from build123d import *

# Parameters (mm, degrees)
SKETCH1_W                = 20
SKETCH1_H                = 60
BOSS_EXTRUDE1_DEPTH      = 15
SKETCH2_W                = 10.25
SKETCH2_H                = 10.1
CUT_EXTRUDE1_DEPTH       = 1
CUT_EXTRUDE1_DEPTH_BACK  = 21
SKETCH3_R                = 4.15
CUT_EXTRUDE2_DEPTH       = 16
BOSS_EXTRUDE2_DEPTH      = 2.5
BOSS_EXTRUDE2_DEPTH_BACK = 22.5
CHAMFER1_SIZE            = 1
CHAMFER1_SIZE2           = 0.577350269
CHAMFER1_PART_2_SIZE     = 1
CHAMFER1_PART_2_SIZE2    = 0.577350269


with BuildPart() as part:
    # Sketch1 → Boss-Extrude1 (new body)
    with BuildSketch(Plane(origin=(0, 0, 0), x_dir=(1, 0, 0), z_dir=(0, 1, 0))):
        Rectangle(SKETCH1_W, SKETCH1_H)
    extrude(amount=BOSS_EXTRUDE1_DEPTH)

    # Sketch2 → Cut-Extrude1 (cut, two sides)
    with BuildSketch(Plane(origin=(10, 0, 0), x_dir=(0, 0, -1), z_dir=(1, 0, 0))) as cut_extrude1_sk:
        with Locations((0, 5.05)):
            Rectangle(SKETCH2_W, SKETCH2_H)
    extrude(amount=CUT_EXTRUDE1_DEPTH, mode=Mode.SUBTRACT)
    extrude(cut_extrude1_sk.sketch, amount=-CUT_EXTRUDE1_DEPTH_BACK, mode=Mode.SUBTRACT)

    # Sketch3 → Cut-Extrude2 (cut, through all)
    with BuildSketch(Plane.XZ):
        with Locations(Location((0, 20, 0), (0, 0, 270))):  # turned: the seam where the file's is
            Circle(SKETCH3_R)
        with Locations(Location((0, -20, 0), (0, 0, 270))):  # turned: the seam where the file's is
            Circle(SKETCH3_R)
    extrude(amount=-CUT_EXTRUDE2_DEPTH, mode=Mode.SUBTRACT)

    # Sketch4 → Boss-Extrude2 (add, two sides)
    with BuildSketch(Plane(origin=(10, 0, 0), x_dir=(0, 0, -1), z_dir=(1, 0, 0))) as boss_extrude2_sk:
        Polygon((-5.125, 0), (-9.975, 0), (-9.975, 15), (9.975, 15), (9.975, 0), (5.125, 0), (5.125, 10.1), (-5.125, 10.1), align=None)
    extrude(amount=BOSS_EXTRUDE2_DEPTH)
    extrude(boss_extrude2_sk.sketch, amount=-BOSS_EXTRUDE2_DEPTH_BACK)

    # Chamfer1
    chamfer1_edges = [part.edges().sort_by_distance(p)[0] for p in [
        (0, 15, 24.15),
    ]]
    chamfer1_side = [part.faces().sort_by_distance(p)[0] for p in [
        (0, 7.5, 24.15),
    ]]
    chamfer(chamfer1_edges, length=CHAMFER1_SIZE, length2=CHAMFER1_SIZE2, reference=chamfer1_side[0])

    # Chamfer1 part 2
    chamfer1_part_2_edges = [part.edges().sort_by_distance(p)[0] for p in [
        (0, 15, -15.85),
    ]]
    chamfer1_part_2_side = [part.faces().sort_by_distance(p)[0] for p in [
        (0, 7.5, -15.85),
    ]]
    chamfer(chamfer1_part_2_edges, length=CHAMFER1_PART_2_SIZE, length2=CHAMFER1_PART_2_SIZE2, reference=chamfer1_part_2_side[0])


solid = part.part
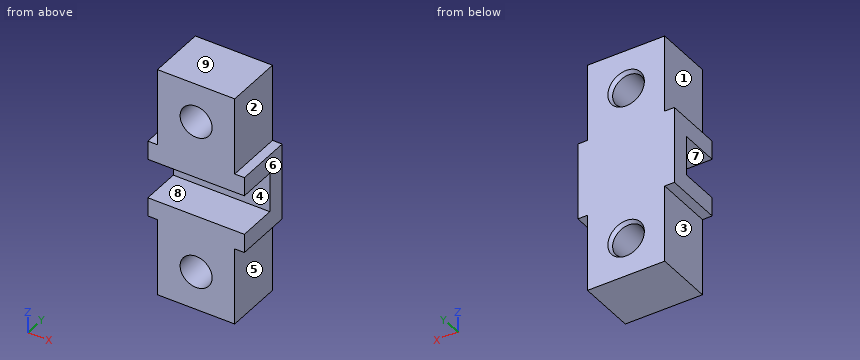
Build history of the part. All positions in model axes, mm. Face numbers are marked on the shaded views. A direction names the side the tool comes from. Round coordinates to 2 decimals unless told otherwise and drop trailing zeros. Write each loop counter-clockwise with the first axis right and the second up, starting at its lowest first coordinate (ties: lowest second). Pieces come first, ordered by that corner, then holes. Notation, with made-up numbers: M -31,-12 L -4,-12 A27 ccw -4,9 Z; hole C 83,66 d2. An arc over 180 degrees is marked long. Answer as a JSON object with one key per item and string values. Group by question number.
(1) Cut at C-C (z = 20). Give the cut face in (x, y), and give its area (3 significant figures).
(2) Drill centre lines: L1, parallel to Z at x = -7.25, y = 2 (3 decimals); L2, parallel to Z at x = 0.5, y = 11.5; L3, parallel to Y at x = -8.75, z = 3. Where is each one in solid material? Low to high.
(3) Mould opens along Z. For the marked faces 6, 7, 8 and 9 say: pulls with the +Z half, pulls with the -Z half, needs draft (parallel to the pull), parting line crosses it, or undercut.
(4) Cut at B-B (y = 8). Give the cut face in (x, z) (3 decimals), and give its area (3 significant figures).
(5) Flat gauge pins, fed straight in: pin 1 (1.5 mm diameter, centred on x = -6.5, z = 18.5, fed in from -Y); pin 2 (5 mm diameter, centred on x = 0, z = -20, fed in from -Y); pin 3 (3 mm diameter, centred on x = -2, z = 1.5, fed in from -Y); pin 4 (1.5 mm diameter, centred on y = 4.5, z = 15.5, fed in from -X). Where does each tip first touch, or does it go through?
(6) Which spindle directions (+Z, -Z, +X, -X, +Y, -Y) get a long thin tool onto all of the face, cutting with end or side? Do the marked faces 1, 2, 3, 4 and 5. Say none if no direction does.
(7) Cut at A-A (x = 0). Give the cut face in (y, z) (3 decimals), and give its area (3 significant figures).
Responses:
{
 "1": {"outline": "M -10,0 L -4.15,0 L -4.15,14 L -4.73,15 L -10,15 Z; M 4.15,0 L 10,0 L 10,15 L 4.73,15 L 4.15,14 Z", "area": "175 mm2"},
 "2": {"L1": "z = -30 to -5.125, 5.125 to 30", "L2": "z = -30 to -24.12, -15.88 to 15.88, 24.12 to 30", "L3": "y = 10.1 to 15"},
 "3": {"face 6": "needs draft", "face 7": "undercut", "face 8": "undercut", "face 9": "pulls with the +Z half"},
 "4": {"outline": "M -12.5,-9.975 L -10,-9.975 L -10,-30 L 10,-30 L 10,-9.975 L 12.5,-9.975 L 12.5,-5.125 L -12.5,-5.125 Z; M -12.5,5.125 L 12.5,5.125 L 12.5,9.975 L 10,9.975 L 10,30 L -10,30 L -10,9.975 L -12.5,9.975 Z; hole C 0,-20 d8.3; hole C 0,20 d8.3", "area": "935 mm2"},
 "5": {"pin 1": "stops at y = 0", "pin 2": "passes through", "pin 3": "stops at y = 10.1", "pin 4": "stops at x = -10"},
 "6": {"face 1": "+Z, -X, +Y, -Y", "face 2": "+Z, +X, +Y, -Y", "face 3": "-Z, -X, +Y, -Y", "face 4": "+X, -X, -Y", "face 5": "-Z, +X, +Y, -Y"},
 "7": {"outline": "M 0,-30 L 15,-30 L 15,-24.727 L 14,-24.15 L 0,-24.15 Z; M 0,-15.85 L 14,-15.85 L 15,-15.273 L 15,15.273 L 14,15.85 L 0,15.85 L 0,5.125 L 10.1,5.125 L 10.1,-5.125 L 0,-5.125 Z; M 0,24.15 L 14,24.15 L 15,24.727 L 15,30 L 0,30 Z", "area": "546 mm2"}
}
